Source: CAD feature listing. Evaluate the final solid. Frame: model axes, mm. A direction names the side the tool comes from. Round coordinates to 2 decimals unless told otherwise and drop trailing zeros. Order: outer loops, then holes, each group sorted by start corner. A loop starts at its lowest first (then second) coordinate and runs counter-clockwise, first axis right, second up. Notation, with made-up numbers: M -29.75,-30.75 L -0.75,-30.75 A23 ccw -0.75,8.25 Z; hole C -3,-20 d1. An arc over 180 degrees is marked long. Use one line per item in the form item = value. Start each with the question number.
Q1. Material intervals for probe 1 along Y at (x, z) = (1, 0); probe 2 along Z at (x, y) = (4, 48); probe 3 along Z at (x, y) = (1.3, -12.5), sorted ascending.
Q2. Pull-direction query (Y, two-part tool) for faces 1 (the flat face through (12, 24, 15)), 2 (the cylindrical face through (1, -85, 0)), 3 (the flat face through (1.7, -100, 0.2)); classes: pulls with the +Y half, pulls with the -Y half, needs draft (parallel to the pull), parting line crosses it, or undercut.
Q3. Contact query for flat-ended pins moving along their axis: pin 1 (0.6 mm diameter, centred on x = 21.5, z = -14, fed in from -Y); pin 2 (10 mm diameter, centred on y = -16.5, z = -10, fed in from +X); pin 3 (8 mm diameter, centred on y = -47, z = 3, fed in from +X). Output: stop coordinate, or through.
Q4. Section C-C (x = 23). Return the cut outline in (y, z).
Q5. Reachability of faces 4 (the flat face through (13, 24, 13)), 5 (the cylindrical face through (1.01, -14.94, 0.54)) from +Z, -Z, +X, -X, +Y, -Y: full face, straight path, thin tool, end or side. Return the list, or none.
Q6. Section B-B (z = 0). Return the cut outline in (x, y).
Q7. Section A-A (y = -12.5). Return the cut outline in (x, z), plus the area to 3 significant figures.
Q8. Section D-D (y = 8.5). Return the cut outline in (x, z), plus the area to 3 significant figures.
Solid Edge part; units mm, degrees
sketch "Sketch1" plane through (0, 0, 0) normal (0, -1, 0) x (1, 0, 0)
  line L0 (0, 15) -> (0, -15)
  line L1 (0, -15) -> (30, -15)
  line L2 (30, -15) -> (30, -13)
  line L3 (30, -13) -> (2, -13)
  line L4 (2, -13) -> (2, 13)
  line L5 (2, 13) -> (30, 13)
  line L6 (30, 13) -> (30, 15)
  line L7 (30, 15) -> (0, 15)
  dimension "D1" = 30
  dimension "D2" = 30
extrude "Protrusion1" add sketch "Sketch1" along normal mid plane 200
sketch "Sketch2" plane through (15, 0, 15) normal (0, 0, 1) x (0, -1, 0)
  line L0 (0, 15) -> (0, -5)
  line L1 (0, -5) -> (100, -5)
  line L2 (100, -5) -> (100, 15)
  line L3 (100, 15) -> (0, 15)
  dimension "D1" = 100
extrude "Cutout1" cut sketch "Sketch2" against normal through all
hole "Hole_1" at (2, -87.5, 0) direction (-1, 0, 0) diameter 5 end up to next
hole "Hole1" at (2, -12.5, 0) direction (-1, 0, 0) diameter 5 end up to next
properties material "Aluminum, 1060"
Results list:
q1.probe_1 = -100 to -90, -85 to -15, -10 to 100
q1.probe_2 = -15 to -13, 13 to 15
q1.probe_3 = -15 to -2.5, 2.5 to 15
q2.face_1 = needs draft
q2.face_2 = undercut
q2.face_3 = pulls with the -Y half
q3.pin_1 = 0
q3.pin_2 = 10
q3.pin_3 = 2
q4.outline = M 0,-15 L 100,-15 L 100,-13 L 0,-13 Z; M 0,13 L 100,13 L 100,15 L 0,15 Z
q5.face_4 = +X, +Y, -Y
q5.face_5 = +X, -X
q6.outline = M 0,-100 L 2,-100 L 2,-90 L 0,-90 Z; M 0,-85 L 2,-85 L 2,-15 L 0,-15 Z; M 0,-10 L 2,-10 L 2,100 L 0,100 Z
q7.outline = M 0,-15 L 10,-15 L 10,-13 L 2,-13 L 2,-2.5 L 0,-2.5 Z; M 0,2.5 L 2,2.5 L 2,13 L 10,13 L 10,15 L 0,15 Z
q7.area = 82.0 mm2
q8.outline = M 0,-15 L 30,-15 L 30,-13 L 2,-13 L 2,13 L 30,13 L 30,15 L 0,15 Z
q8.area = 172 mm2
